Could you check a few things on this model? Use its own coordinates, in mm. Face numbers are marked on the shaded views. A direction names the side the tool comes from. Coordinates: 2 decimals unless noted, no trailing zeros. Order: outer loops, then holes, each group sorted by start corner. A loop starts at its lowest first (then second) coordinate and runs counter-clockwise, first axis right, second up. Notation, with made-up numbers: (-36, -22) - (-9, -22) arc R22 cw to (-9, -7) - close; hole circle Ø5 at (55, -37.75). An arc over 180 degrees is marked (long way). One line per item, written item: value.
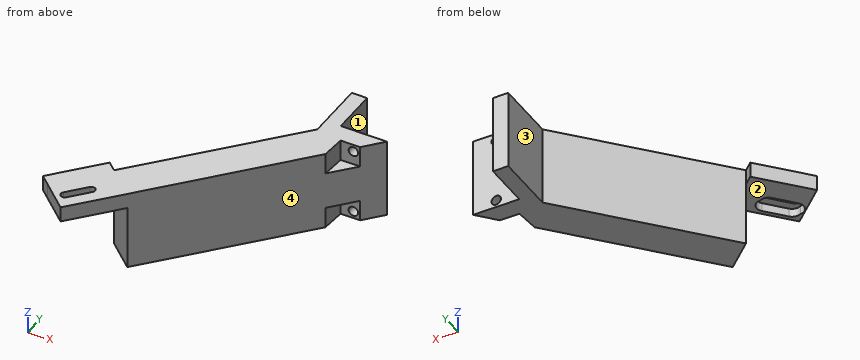
Autodesk Inventor part; units mm, degrees
ref_plane "Work Plane2" through (-4.445, -9.144, -33.02) normal (0, 0, -1) x (0, 1, 0)
ref_plane "YZ Plane" through (0, 0, 0) normal (1, 0, 0) x (0, 1, 0)
ref_plane "XZ Plane" through (0, 0, 0) normal (0, 1, 0) x (-1, 0, 0)
ref_plane "Work Plane1" through (0, 0, 0) normal (0, 0, 1) x (1, 0, 0)
sketch "Sketch1" plane through (0, 0, 0) normal (0, 0, 1) x (1, 0, 0)
  line L0 (4.129202, -9.5377) -> (6.406797, -9.5377) construction
  line L1 (9.525, -8.41296) -> (9.525, -7.435497) construction
  line L2 (-6.406797, 9.5123) -> (-4.129202, 9.5123) construction
  line L3 (-9.525, 4.116502) -> (-9.525, 6.394097) construction
  line L4 (9.314549, -9.373063) -> (-73.965447, -101.864868) construction
  line L5 (9.166309, -9.5377) -> (-73.965447, -101.864868)
  line L6 (-73.965447, -101.864868) -> (-85.121243, -91.820144)
  line L7 (6.33881, 9.756536) -> (-85.121243, -91.820144) construction
  line L8 (9.166309, -9.5377) -> (-9.997679, -9.5377)
  line L9 (-9.997679, -9.5377) -> (-9.997679, 9.756536)
  line L10 (-9.997679, 9.756536) -> (-16.347679, 9.756536)
  line L11 (-16.347679, 9.756536) -> (-16.347679, -15.439362)
  line L12 (-16.347679, -15.439362) -> (-85.121243, -91.820144)
  point P0 (0, 0)
  dimension "d0" = 124.46
  dimension "d1" = 48
  dimension "d5" = 6.35
ref_plane "Work Plane2" through (-4.445, -9.144, -33.02) normal (0, 0, -1) x (0, 1, 0)
extrude "Extrusion1" add sketch "Sketch1" against normal up to surface (33.02 mm away)
sketch "Sketch2" plane through (-73.965447, -101.864868, -33.02) normal (-0.6691306, -0.7431448, 0) x (0.7431448, -0.6691306, 0)
  line L0 (0, 33.02) -> (0, 0)
  line L1 (-15.011605, 33.02) -> (-15.011605, 0)
  line L2 (0, 0) -> (-15.011605, 0)
  line L3 (-15.011605, 0) -> (-15.011605, 26.67)
  line L4 (-15.011605, 26.67) -> (0, 26.67)
  line L5 (0, 26.67) -> (0, 0)
  line L6 (-15.011605, 33.02) -> (0, 33.02)
  point P0 (-13.193862, 33.02)
  dimension "d19" = 6.35
extrude "Extrusion2" cut sketch "Sketch2" against normal blind 25.4 contours L0 L2 L1 L4
sketch "Sketch3" plane through (-73.965447, -101.864868, -6.35) normal (0, 0, -1) x (-0.7431448, 0.6691306, 0)
  line L0 (19.8882, 12.0904) -> (19.8882, 3.175) construction
  line L1 (0, 25.4) -> (15.011605, 25.4) construction
  line L2 (15.011605, 0) -> (0, 0) construction
  line L3 (0, 0) -> (19.8882, 0) construction
  line L4 (19.8882, 0) -> (19.8882, 25.4) construction
  line L5 (19.8882, 25.4) -> (0, 25.4) construction
  line L6 (0, 25.4) -> (0, 0) construction
  line L7 (15.011605, 0) -> (19.8882, 0)
  line L8 (19.8882, 0) -> (19.8882, 25.4)
  line L9 (19.8882, 25.4) -> (15.011605, 25.4)
  line L10 (15.011605, 25.4) -> (15.011605, 0)
  point P0 (13.193862, 125.192894)
extrude "Extrusion3" add sketch "Sketch3" against normal up to surface (6.35 mm away)
sketch "Sketch4" plane through (0, 0, 0) normal (0, 0, 1) x (1, 0, 0)
  circle A0 centre (-72.965209, -90.773771) radius 1.1938 construction
  circle A1 centre (-65.459407, -96.637946) radius 1.1938 construction
  line L0 (-72.965209, -90.773771) -> (-64.699827, -81.594134) construction
  line L1 (-88.74526, -88.557064) -> (-71.749342, -69.681186) construction
  line L2 (-72.965209, -90.773771) -> (-77.668593, -95.997407) construction
  line L3 (-76.364393, -94.548947) -> (-69.566026, -86.998595) construction
  line L4 (-75.194088, -95.602693) -> (-68.395721, -88.052342)
  line L5 (-70.73633, -85.944848) -> (-77.534697, -93.4952)
  arc A2 (-77.534697, -93.4952) -> (-75.194088, -95.602693) centre (-76.364393, -94.548947) ccw
  arc A3 (-68.395721, -88.052342) -> (-70.73633, -85.944848) centre (-69.566026, -86.998595) ccw
  line L6 (-65.459407, -96.637946) -> (-57.773123, -88.101463) construction
  line L7 (-73.965447, -101.864868) -> (9.166309, -9.5377) construction
  line L8 (-65.459407, -96.637946) -> (-69.368096, -100.978985) construction
  line L9 (-68.85859, -100.413122) -> (-62.060223, -92.862771) construction
  line L10 (-67.688286, -101.466869) -> (-60.889919, -93.916518)
  line L11 (-63.230528, -91.809024) -> (-70.028895, -99.359375)
  arc A4 (-70.028895, -99.359375) -> (-67.688286, -101.466869) centre (-68.85859, -100.413122) ccw
  arc A5 (-60.889919, -93.916518) -> (-63.230528, -91.809024) centre (-62.060223, -92.862771) ccw
  point P0 (0, 0)
  dimension "d13" = 5.08
  dimension "d14" = 3.1496
  dimension "d15" = 5.08
  dimension "d16" = 3.1496
extrude "Extrusion4" cut sketch "Sketch4" against normal through all
sketch "Sketch5" plane through (-73.965447, -101.864868, -6.35) normal (0, 0, -1) x (-0.7431448, 0.6691306, 0)
  arc A0 (6.7564, 14.73835) -> (3.6068, 14.73835) centre (5.1816, 14.73835) ccw
  arc A1 (3.6068, 4.57835) -> (6.7564, 4.57835) centre (5.1816, 4.57835) ccw
  line L0 (5.1816, 14.73835) -> (5.1816, 4.57835) construction
  line L1 (1.6256, 14.73835) -> (1.6256, 4.57835)
  line L2 (8.7376, 4.57835) -> (8.7376, 14.73835)
  arc A2 (8.7376, 14.73835) -> (1.6256, 14.73835) centre (5.1816, 14.73835) ccw
  arc A3 (1.6256, 4.57835) -> (8.7376, 4.57835) centre (5.1816, 4.57835) ccw
  arc A4 (8.252871, 13.991581) -> (5.103271, 13.991581) centre (6.678071, 13.991581) ccw
  arc A5 (5.103271, 3.831581) -> (8.252871, 3.831581) centre (6.678071, 3.831581) ccw
  line L3 (6.678071, 13.991581) -> (6.678071, 3.831581) construction
  line L4 (3.122071, 13.991581) -> (3.122071, 3.831581)
  line L5 (10.234071, 3.831581) -> (10.234071, 13.991581)
  arc A6 (10.234071, 13.991581) -> (3.122071, 13.991581) centre (6.678071, 13.991581) ccw
  arc A7 (3.122071, 3.831581) -> (10.234071, 3.831581) centre (6.678071, 3.831581) ccw
  point P0 (13.193862, 125.192894)
  point P1 (5.1816, 9.65835)
  point P2 (6.678071, 8.911581)
  dimension "d20" = 7.112
  dimension "d21" = 7.112
sketch "Sketch5 outline for Extrusion5" plane through (-73.965447, -101.864868, -6.35) normal (0, 0, -1) x (-0.7431448, 0.6691306, 0)
  line L0 (10.234071, 3.831581) -> (10.234071, 13.991581)
  arc A0 (10.234071, 13.991581) -> (7.473106, 17.457566) centre (6.678071, 13.991581) ccw
  arc A1 (7.473106, 17.457566) -> (1.6256, 14.73835) centre (5.1816, 14.73835) ccw
  line L1 (1.6256, 14.73835) -> (1.6256, 4.57835)
  arc A2 (1.6256, 4.57835) -> (4.386565, 1.112364) centre (5.1816, 4.57835) ccw
  arc A3 (4.386565, 1.112364) -> (10.234071, 3.831581) centre (6.678071, 3.831581) ccw
extrude "Extrusion5" cut sketch "Sketch5 outline for Extrusion5" against normal blind 3.556
sketch "Sketch6" plane through (-9.997679, -9.5377, 0) normal (0, 1, 0) x (1, 0, 0)
  arc A0 (9.506526, 4.79213) -> (10.740649, 4.300966) centre (9.523849, 3.039616) ccw construction
  arc A1 (9.506526, 31.732899) -> (10.740649, 31.241734) centre (9.523849, 29.980384) ccw construction
  circle A2 centre (9.523849, 29.980384) radius 1.9685
  circle A3 centre (9.523849, 3.039616) radius 1.9685
  point P0 (9.997679, 0)
  dimension "d24" = 3.937
  dimension "d25" = 3.937
extrude "Extrusion6" cut sketch "Sketch6" against normal through all
sketch "Sketch7" plane through (9.166309, -9.5377, 0) normal (0.7431448, -0.6691306, 0) x (0, 0, -1)
  line L0 (33.02, -98.838459) -> (33.02, 0) construction
  line L1 (33.02, -9.525) -> (0, -9.525) construction
  point P0 (0, 0.954435)
sketch "Sketch8" plane through (9.166309, -9.5377, -33.02) normal (0, 0, -1) x (-1, 0, 0)
  line L0 (11.608639, 0) -> (11.608639, -12.892699) construction
  line L1 (66.135838, -73.451289) -> (0, 0) construction
  line L2 (11.608639, -7.62) -> (6.861079, -7.62) construction
  line L3 (0, 0) -> (19.163987, 0) construction
  line L4 (7.671639, 0) -> (7.671639, -8.520218) construction
  line L5 (14.910639, 0) -> (14.910639, -14.251905) construction
  line L6 (6.861079, -7.62) -> (14.910639, -7.62)
  line L7 (83.131755, -92.327168) -> (0, 0)
  line L8 (15.69062, -17.426199) -> (6.861079, -7.62)
  line L9 (15.69062, -17.426199) -> (14.910639, -7.62)
  point P0 (9.166309, 9.5377)
  dimension "d28" = 7.62
  dimension "d29" = 3.302
extrude "Extrusion7" cut sketch "Sketch8" against normal blind 8.763
sketch "Sketch9" plane through (0, 0, 0) normal (0, 0, 1) x (1, 0, 0)
  line L0 (2.30523, -17.1577) -> (-5.74433, -17.1577) construction
  line L1 (-5.74433, -17.1577) -> (-6.524312, -26.963899) construction
  line L2 (2.30523, -17.1577) -> (-6.524312, -26.963899)
  line L3 (-73.965447, -101.864868) -> (9.166309, -9.5377)
  line L4 (2.30523, -17.1577) -> (-5.74433, -17.1577)
  line L5 (-5.2705, -26.963899) -> (-5.2705, -17.1577)
  point P0 (0, 0)
sketch "Sketch9 outline for Extrusion8" plane through (0, 0, 0) normal (0, 0, 1) x (1, 0, 0)
  line L0 (-6.524312, -26.963899) -> (2.30523, -17.1577)
  line L1 (-5.74433, -17.1577) -> (-6.524312, -26.963899)
  line L2 (2.30523, -17.1577) -> (-5.74433, -17.1577)
extrude "Extrusion8" cut sketch "Sketch9 outline for Extrusion8" against normal blind 8.763
properties part number "arm stop"
Item 1: If I drill on probe 1 along X at (y, z) = (3.5, -5); probe 2 along X at (y, z) = (-71, -21.5); probe 3 along Y at (x, z) = (-0.5, -14.5), over which ranges is the centre line in solid material (lowest first)?
Conclusion:
probe 1: -16.35 to -10
probe 2: -66.37 to -46.17
probe 3: -20.27 to -9.54
Item 2: For the marked faces 1, 2, 3 and 4, which set-ups out of +Z, -Z, +X, -X, +Y, -Y let a thin tool reach every point of the face, with its end or its side?
Conclusion:
face 1: +Z, -Z, +X, +Y
face 2: -Z, -X, -Y
face 3: +Z, -Z, -X, +Y
face 4: +Z, -Z, +X, -Y
Item 3: I want a section at A-A on z = -18. Please give me the cut outline in (x, y).
Conclusion:
outline: (-68.12, -72.94) - (-56.97, -82.99) - (9.17, -9.54) - (-10, -9.54) - (-10, 9.76) - (-16.35, 9.76) - (-16.35, -15.44) - close
Item 4: I'm going to push flat-ended pins straight in: pin 1 Ø4 at (x, z) = (-3, -29.5) entering from -Y; pin 2 Ø9.5 at (x, z) = (3, -16.5) entering from +Y; pin 3 Ø2 at (x, z) = (-60, -23) entering from +Y. Where does each tip first touch, or does it pass through?
Conclusion:
pin 1: y = -17.16
pin 2: y = -9.54
pin 3: y = -62.81
Item 5: I want a section at C-C on x = -48. Please give me the cut outline in (y, z), then the cut area to 3 significant figures.
Conclusion:
outline: (-73.03, -33.02) - (-50.59, -33.02) - (-50.59, 0) - (-73.03, 0) - close
area: 741 mm²
Item 6: I want a section at B-B on y = -23. Please give me the cut outline in (x, z).
Conclusion:
outline: (-23.16, -33.02) - (-6.21, -33.02) - (-6.21, -24.26) - (-2.96, -24.26) - (-2.96, -8.76) - (-6.21, -8.76) - (-6.21, 0) - (-23.16, 0) - close
